Job drawing, mm, ordinate dimensions from the low corner. One solid piece. Round coordinates to 2 decimals unless told otherwise and drop trailing zeros. Order: outer loops, then holes, each group sorted by start corner. A loop starts at its lowest first (then second) coordinate and runs counter-clockwise, first axis right, second up. Notation, with made-up numbers: (62, 45) -> (111, 45) arc R11 cw to (111, 66) -> close; hole circle Ø7 at (55, 87). An arc over 180 degrees is marked (long way). Return JSON: item names as keys, results as strings. Group by question number.
Q1. Cut at A-A (y = 10.5). Write the cut outline in (x, z), then the cut area to 3 significant figures.
Q2. Flat gauge pins, fed straight in: pin 1 (0.9 mm diameter, centred on y = 1.5, z = 1.5, fed in from -X); pin 2 (1.5 mm diameter, centred on y = 18, z = 1, fed in from -X); pin 3 (0.9 mm diameter, centred on x = 79.5, z = 2, fed in from +Y); pin 4 (0.9 mm diameter, centred on x = 104.5, z = 1, fed in from -Y). Where does each tip first touch, or does it go through?
Q3. Cut at C-C (x = 74.5). Write the cut outline in (y, z).
Q4. Probe line 1 along X through (y, z) = (30, 2.1); line 2 along X through (y, z) = (13, 2.1); line 3 along X through (y, z) = (21, 2.55). List the from-to ranges inside material, lowest first.
Q5. Cut at B-B (z = 2.3). Count the separate pieces of the cut face and the enclosed holes in it, then the cut area to 3 significant figures.
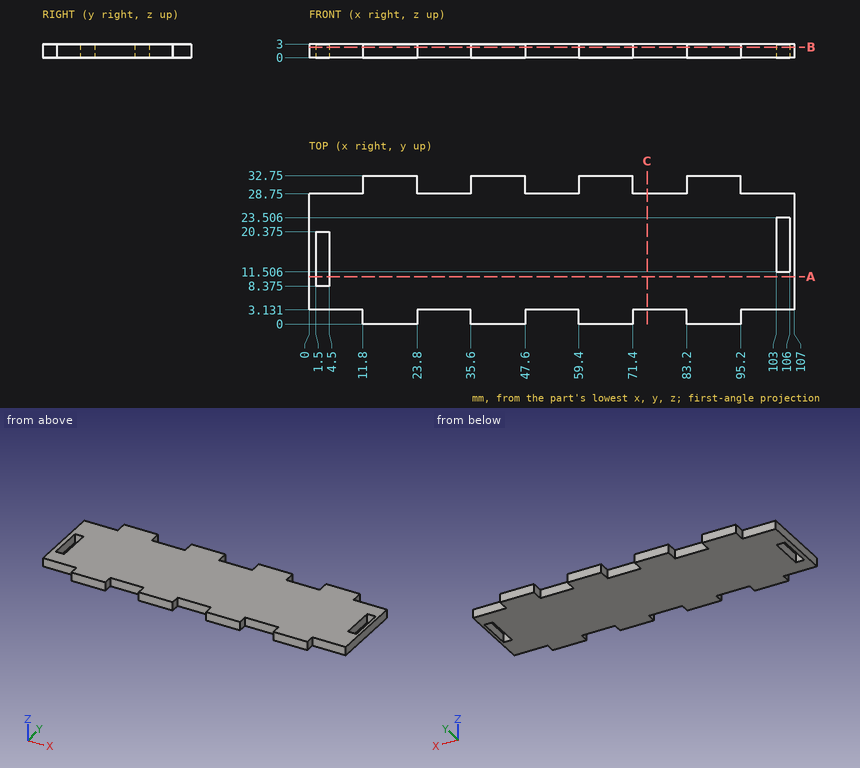
Solution:
{
 "1": {"outline": "(0, 0) -> (1.5, 0) -> (1.5, 3) -> (0, 3) -> close; (4.5, 0) -> (107, 0) -> (107, 3) -> (4.5, 3) -> close", "area": "312 mm²"},
 "2": {"pin 1": "stops at x = 11.8", "pin 2": "stops at x = 0", "pin 3": "stops at y = 28.75", "pin 4": "stops at y = 3.13"},
 "3": {"outline": "(3.13, 0) -> (28.75, 0) -> (28.75, 3) -> (3.13, 3) -> close"},
 "4": {"line 1": "x = 11.8 to 23.8, 35.6 to 47.6, 59.4 to 71.4, 83.2 to 95.2", "line 2": "x = 0 to 1.5, 4.5 to 103, 106 to 107", "line 3": "x = 0 to 103, 106 to 107"},
 "5": {"separate pieces": "1", "enclosed holes": "2", "area": "3,010 mm²"}
}
